Input: part model. Units: mm. Frame: model coordinates. A direction names the side the tool comes from. Give positions to 0.01 mm unless a question says otherwise; leave off trailing zeros. Write each loop counter-clockwise with the first axis right and the second up, starting at its lowest first coordinate (ties: lowest second). Pieces come first, ordered by that corner, then holes. Notation, with made-up numbers: (-4.5, 88) - (2.5, 88) arc R13 cw to (2.5, 93) - close; hole circle Ø3 at (-25, 21). An arc over 180 degrees is marked (long way). Use a Markdown table: item, result. Add a question column.
1. Section query D-D, the plane x = 1.25. Return loops of the section in (y, z), plus the area to 3 significant figures.
2. Material intervals for probe 1 along Z at (x, y) = (-1.25, -1); probe 2 along Y at (x, z) = (0, 1.75); probe 3 along Z at (x, y) = (2, -10.25), sorted ascending.
3. Mould query, pull axis X, two halves, no side actions, for faces 1 (the cylindrical face through (-0.46, 3.47, 1.9)), 2 (the cylindrical face through (2.499, -14.715, 3.01)), 3 (the cylindrical face through (-0.29, 2.23, 1.48)), 4 (the flat face through (0, 0, 3)). Classes: released by +X, released by -X, zero draft, split by the parting line, or undercut.
4. Section query B-B, the plane x = 0. Return loops of the section in (y, z).
5. Section query A-A, the plane z = 2.8. Return loops of the section in (x, y), plus the area to 3 significant figures.
6. Set-up query: faces 5 (the flat face through (0, 0, 3.85)), 6 (the flat face through (-2.5, -8, 3)), 7 (the flat face through (2.8, -8, 3)). Return all of +Z, -Z, +X, -X, +Y, -Y with unobstructed straight access to the full face (end or side cutting, diameter ignored); none if empty.
7. Section query C-C, the plane y = 0. Return loops of the section in (x, z), plus the area to 4 significant figures.
8. Pin query (flat end, axial travel): pin 1 (4 mm diameter, centred on x = 1, y = -10.5, fed in from -Z); pin 2 (1.3 mm diameter, centred on x = 1, y = -0.5, fed in from -Z); pin 3 (1.2 mm diameter, centred on y = -10.5, z = 3.5, fed in from +X). Return the tip coordinate at first contact, or that it passes through.
```python
from build123d import *

# Parameters (mm, degrees)
CYLINDER006_R     = 2.25
CYLINDER006_DEPTH = 3
BOX001_W          = 5.3
BOX001_H          = 13.5
BOX001_DEPTH      = 1.5
FILLET_R          = 1
CYLINDER005_R     = 3.5
CYLINDER005_DEPTH = 3.85


with BuildPart() as cylinder006:
    # Cylinder006 → Cylinder006 (new body)
    with BuildSketch(Plane.XY):
        Circle(CYLINDER006_R)
    extrude(amount=CYLINDER006_DEPTH)


with BuildPart() as fillet_body:
    # Box001 → Box001 (new body)
    with BuildSketch(Plane(origin=(-2.5, -15, 2.25), x_dir=(1, 0, 0), z_dir=(0, 0, 1))):
        with Locations((2.65, 6.75)):
            Rectangle(BOX001_W, BOX001_H)
    extrude(amount=BOX001_DEPTH)

    # Fillet
    fillet_edges = [fillet_body.edges().sort_by_distance(p)[0] for p in [
        (-2.5, -15, 3),
        (2.8, -15, 3),
    ]]
    fillet(fillet_edges, radius=FILLET_R)


with BuildPart() as servoarmsingle:
    # Cylinder005 → Cylinder005 (new body)
    with BuildSketch(Plane.XY):
        Circle(CYLINDER005_R)
    extrude(amount=CYLINDER005_DEPTH)

    # Fusion003: union Fillet body
    add(fillet_body.part)

    # Cut001: cut Cylinder006
    add(cylinder006.part, mode=Mode.SUBTRACT)


solid = servoarmsingle.part
```
Result sheet:
| question | item | result |
|---|---|---|
| 1 | outline | (-15, 2.25) - (-3.27, 2.25) - (-3.27, 0) - (-1.87, 0) - (-1.87, 3) - (1.87, 3) - (1.87, 0) - (3.27, 0) - (3.27, 3.85) - (-3.27, 3.85) - (-3.27, 3.75) - (-15, 3.75) - close |
| 1 | area | 31.5 mm² |
| 2 | probe 1 | z = 3 to 3.85 |
| 2 | probe 2 | y = -3.5 to -2.25, 2.25 to 3.5 |
| 2 | probe 3 | z = 2.25 to 3.75 |
| 3 | face 1 | split by the parting line |
| 3 | face 2 | released by +X |
| 3 | face 3 | undercut |
| 3 | face 4 | undercut |
| 4 | outline | (-15, 2.25) - (-3.5, 2.25) - (-3.5, 0) - (-2.25, 0) - (-2.25, 3) - (2.25, 3) - (2.25, 0) - (3.5, 0) - (3.5, 3.85) - (-3.5, 3.85) - (-3.5, 3.75) - (-15, 3.75) - close |
| 5 | outline | (-2.5, -14) arc R1 ccw to (-1.5, -15) - (1.8, -15) arc R1 ccw to (2.8, -14) - (2.8, -2.1) arc R3.5 ccw (long way) to (-2.5, -2.45) - close; hole circle Ø4.5 at (0, 0) |
| 5 | area | 85.1 mm² |
| 6 | face 5 | +Z, +X, -X, +Y, -Y |
| 6 | face 6 | +Z, -Z, -X, -Y |
| 6 | face 7 | +Z, -Z, +X, -Y |
| 7 | outline | (-3.5, 0) - (-2.25, 0) - (-2.25, 3) - (2.25, 3) - (2.25, 0) - (3.5, 0) - (3.5, 3.85) - (-3.5, 3.85) - close |
| 7 | area | 13.45 mm² |
| 8 | pin 1 | stops at z = 2.25 |
| 8 | pin 2 | stops at z = 3 |
| 8 | pin 3 | stops at x = 2.8 |
